Input: part model. Units: mm. Frame: model coordinates. A direction names the side the tool comes from. Round coordinates to 2 decimals unless told otherwise and drop trailing zeros. Order: outer loops, then holes, each group sorted by start corner. A loop starts at its lowest first (then second) coordinate and runs counter-clockwise, first axis right, second up. Notation, with made-up numbers: (73, 61.25) -> (128, 61.25) arc R22 cw to (128, 97.25) -> close; hole circle Ø11 at (-17.75, -11.5). An arc over 180 degrees is marked (long way). Use a Markdown table: item, result.
from build123d import *

# Parameters (mm, degrees)
F1_DEPTH = 1200
F3_D     = 8
F4_R     = 2


# Not quite as in the source:
# - a feature names something its author has since deleted; it is built from what else it names


with BuildPart() as f1:
    # F0 (on Right) → F1 (new body)
    with BuildSketch(Plane.YZ):
        Polygon((-18.8378913403, 427.8021101952), (-18.8378913403, 404.8021101952), (-16.8378913403, 404.8021101952), (-16.8378913403, 429.8021101952), (-56.8378913403, 429.8021101952), (-56.8378913403, 79.8021101952), (-29.8378913403, 79.8021101952), (-29.8378913403, 53.8021101952), (-27.8378913403, 53.8021101952), (-27.8378913403, 81.8021101952), (-54.8378913403, 81.8021101952), (-54.8378913403, 427.8021101952), align=None)
    extrude(amount=F1_DEPTH)

    # F3 (through all)
    with Locations(Plane.XZ.offset(29.8378913403)):
        with Locations((433, 66.8021101952), (767, 66.8021101952), (1100, 66.8021101952), (100, 66.8021101952)):
            Hole(F3_D / 2)

    # F4
    f4_edges = [f1.edges().sort_by_distance(p)[0] for p in [
        (600, -56.837891, 429.80211),
        (600, -16.837891, 429.80211),
        (600, -56.837891, 79.80211),
        (600, -27.837891, 81.80211),
        (600, -54.837891, 81.80211),
        (600, -29.837891, 79.80211),
        (600, -18.837891, 427.80211),
        (600, -54.837891, 427.80211),
    ]]
    fillet(f4_edges, radius=F4_R)


solid = f1.part
1) Contact query for flat-ended pins moving along their axis: P1, Ø6.5, axis at x = 433, z = 66.8, coming from the -Y side; P2, Ø21, axis at x = 404, z = 68, coming from the +Y side; P3, Ø18.5, axis at x = 565.5, y = -48.5, coming from the -Z side; P4, Ø8, axis at x = 741.5, z = 312.5, coming from the +Y side. Output: stop coordinate, or through.
Answer key:
| item | result |
|---|---|
| P1 | passes through |
| P2 | stops at y = -27.84 |
| P3 | stops at z = 79.8 |
| P4 | stops at y = -54.84 |
2) Cut plane C-C on z = 288.5. Return loops of the section in (x, y), and give its area (3 significant figures).
Answer key:
| item | result |
|---|---|
| outline | (0, -56.84) -> (1200, -56.84) -> (1200, -54.84) -> (0, -54.84) -> close |
| area | 2,400 mm^2 |
3) Cut plane A-A on y = -41.5. Return loops of the section in (x, z).
Answer key:
| item | result |
|---|---|
| outline | (0, 79.8) -> (1200, 79.8) -> (1200, 81.8) -> (0, 81.8) -> close; (0, 427.8) -> (1200, 427.8) -> (1200, 429.8) -> (0, 429.8) -> close |
4) Ray query, probe 1 along Z at (x, y) = (100, -29); probe 2 along Z at (x, y) = (433, -29.3); probe 3 along Z at (x, y) = (491, -46). Return the intervals inside material, ascending.
Answer key:
| item | result |
|---|---|
| probe 1 | z = 53.8 to 62.8, 70.8 to 81.62, 427.8 to 429.8 |
| probe 2 | z = 53.8 to 62.8, 70.8 to 81.73, 427.8 to 429.8 |
| probe 3 | z = 79.8 to 81.8, 427.8 to 429.8 |
5) Cut plane B-B on x = 248.5. Return loops of the section in (y, z).
Answer key:
| item | result |
|---|---|
| outline | (-56.84, 81.8) arc R2 ccw to (-54.84, 79.8) -> (-31.84, 79.8) arc R2 cw to (-29.84, 77.8) -> (-29.84, 53.8) -> (-27.84, 53.8) -> (-27.84, 79.8) arc R2 ccw to (-29.84, 81.8) -> (-52.84, 81.8) arc R2 cw to (-54.84, 83.8) -> (-54.84, 425.8) arc R2 cw to (-52.84, 427.8) -> (-20.84, 427.8) arc R2 cw to (-18.84, 425.8) -> (-18.84, 404.8) -> (-16.84, 404.8) -> (-16.84, 427.8) arc R2 ccw to (-18.84, 429.8) -> (-54.84, 429.8) arc R2 ccw to (-56.84, 427.8) -> close |
6) Set-up query: faces 5 (the face through (592, -43, 79.802)), 6 (the face through (592, -41, 81.802)), 7 (the face through (592, -27.838, 67)). Return all of +Z, -Z, +X, -X, +Y, -Y with unobstructed straight access to the full face (end or side cutting, diameter ignored); none if empty.
Answer key:
| item | result |
|---|---|
| face 5 | -Z, +X, -X, -Y |
| face 6 | +X, -X, +Y |
| face 7 | -Z, +X, -X, +Y |
7) Draft query along Y for faces 1 (the face through (592, -16.838, 416)), 2 (the face through (592, -18.838, 415)), 3 (the face through (592, -29.838, 66)), 4 (the face through (0, -56, 243)). Return one class per face: released by +Y, released by -Y, zero draft, split by the parting line, or undercut.
Answer key:
| item | result |
|---|---|
| face 1 | released by +Y |
| face 2 | undercut |
| face 3 | released by -Y |
| face 4 | zero draft |
